Can you work these out from the model? Positions are in its coordinate system, mm. Round coordinates to 2 decimals unless told otherwise and drop trailing zeros. Loops run counter-clockwise (first coordinate to the right, second up) from the corner with the lowest first, then second, coordinate; pieces in that order, holes last. Notation, with made-up numbers: M 13,88 L 58,88 A20 cw 58,102 Z; hole C -35,46.25 d8. An arc over 180 degrees is marked long. Return JSON: item names as keys, results as strings.
```python
from build123d import *

# Parameters (mm, degrees)
ESQUISSE1_R        = 6.75
ESQUISSE1_R_2      = 41.5
ESQUISSE1_W        = 40
ESQUISSE1_H        = 80
BOSS_EXTRU_1_DEPTH = 10
CONG_1_R           = 10


with BuildPart() as part:
    # Esquisse1 → Boss.-Extru.1 (new body)
    with BuildSketch(Plane(origin=(0, 0, 0), x_dir=(0, 0, -1), z_dir=(1, 0, 0))):
        with BuildLine():
            ThreePointArc((229.796105276, 60), (0, 237.5), (-229.796105276, 60))
            ThreePointArc((-229.796105276, 60), (-231.618451309, 52.527545282), (-233.197877349, 45))
            ThreePointArc((-233.197877349, 45), (-237.5, 0), (-233.197877349, -45))
            ThreePointArc((-233.197877349, -45), (-231.618451309, -52.527545282), (-229.796105276, -60))
            ThreePointArc((-229.796105276, -60), (0, -237.5), (229.796105276, -60))
            ThreePointArc((229.796105276, -60), (231.618451309, -52.527545282), (233.197877349, -45))
            ThreePointArc((233.197877349, -45), (236.422022949, -22.602589781), (237.5, 0))
            ThreePointArc((237.5, 0), (236.422022949, 22.602589781), (233.197877349, 45))
            ThreePointArc((233.197877349, 45), (231.618451309, 52.527545282), (229.796105276, 60))
        make_face()
        with Locations((-158.391918986, -158.391918986)):
            Circle(ESQUISSE1_R, mode=Mode.SUBTRACT)
        with Locations((-85.72108885, -206.949015283)):
            Circle(ESQUISSE1_R, mode=Mode.SUBTRACT)
        with Locations((-206.949015283, -85.72108885)):
            Circle(ESQUISSE1_R, mode=Mode.SUBTRACT)
        with Locations((-224, 0)):
            Circle(ESQUISSE1_R, mode=Mode.SUBTRACT)
        with Locations((-53, -98.5)):
            Circle(ESQUISSE1_R, mode=Mode.SUBTRACT)
        with Locations((0, -224)):
            Circle(ESQUISSE1_R, mode=Mode.SUBTRACT)
        with Locations((85.72108885, -206.949015283)):
            Circle(ESQUISSE1_R, mode=Mode.SUBTRACT)
        with Locations((158.391918986, -158.391918986)):
            Circle(ESQUISSE1_R, mode=Mode.SUBTRACT)
        with Locations((0, -98.5)):
            Circle(ESQUISSE1_R_2, mode=Mode.SUBTRACT)
        with Locations((53, -98.5)):
            Circle(ESQUISSE1_R, mode=Mode.SUBTRACT)
        with Locations((206.949015283, -85.72108885)):
            Circle(ESQUISSE1_R, mode=Mode.SUBTRACT)
        with Locations((-150, 0)):
            Rectangle(ESQUISSE1_W, ESQUISSE1_H, mode=Mode.SUBTRACT)
        with Locations((-206.949015283, 85.72108885)):
            Circle(ESQUISSE1_R, mode=Mode.SUBTRACT)
        with BuildLine():
            Line((-20, 60), (-159.059737206, 60))
            ThreePointArc((-159.059737206, 60), (-104.766475875, 133.880489739), (-20, 168.819430161))
            Line((-20, 168.819430161), (-20, 60))
        make_face(mode=Mode.SUBTRACT)
        with Locations((-158.391918986, 158.391918986)):
            Circle(ESQUISSE1_R, mode=Mode.SUBTRACT)
        with Locations((-85.72108885, 206.949015283)):
            Circle(ESQUISSE1_R, mode=Mode.SUBTRACT)
        with BuildLine():
            Line((159.059737206, 60), (20, 60))
            Line((20, 60), (20, 168.819430161))
            ThreePointArc((20, 168.819430161), (104.766475875, 133.880489739), (159.059737206, 60))
        make_face(mode=Mode.SUBTRACT)
        with Locations((150, 0)):
            Rectangle(ESQUISSE1_W, ESQUISSE1_H, mode=Mode.SUBTRACT)
        with Locations((224, 0)):
            Circle(ESQUISSE1_R, mode=Mode.SUBTRACT)
        with Locations((206.949015283, 85.72108885)):
            Circle(ESQUISSE1_R, mode=Mode.SUBTRACT)
        with Locations((0, 224)):
            Circle(ESQUISSE1_R, mode=Mode.SUBTRACT)
        with Locations((85.72108885, 206.949015283)):
            Circle(ESQUISSE1_R, mode=Mode.SUBTRACT)
        with Locations((158.391918986, 158.391918986)):
            Circle(ESQUISSE1_R, mode=Mode.SUBTRACT)
    extrude(amount=BOSS_EXTRU_1_DEPTH)

    # Cong_1
    cong_1_edges = [part.edges().sort_by_distance(p)[0] for p in [
        (5, 60, -20),
        (5, 60, -159.059737206),
        (5, 168.819430161, -20),
        (5, 60, 159.059737206),
        (5, 60, 20),
        (5, 168.819430161, 20),
    ]]
    fillet(cong_1_edges, radius=CONG_1_R)


solid = part.part
```
Q1. Suppose I cut it at B-B, the plane y = -224. Please give me the cut outline in (x, z).
Results:
{"outline": "M 0,-78.93 L 10,-78.93 L 10,-6.75 L 0,-6.75 Z; M 0,6.75 L 10,6.75 L 10,78.93 L 0,78.93 Z"}
Q2. Suppose I cut it at C-C, the plane z = 53. Please give me the cut outline in (x, y), plus the area to 3 significant figures.
Results:
{"outline": "M 0,-231.51 L 10,-231.51 L 10,-105.25 L 0,-105.25 Z; M 0,-91.75 L 10,-91.75 L 10,60 L 0,60 Z; M 0,161.53 L 10,161.53 L 10,231.51 L 0,231.51 Z", "area": "3,480 mm2"}
Q3. Suppose I cut it at A-A, the plane z = 0. Please give me the cut outline in (x, y), plus the area to 3 significant figures.
Results:
{"outline": "M 0,-237.5 L 10,-237.5 L 10,-230.75 L 0,-230.75 Z; M 0,-217.25 L 10,-217.25 L 10,-140 L 0,-140 Z; M 0,-57 L 10,-57 L 10,217.25 L 0,217.25 Z; M 0,230.75 L 10,230.75 L 10,237.5 L 0,237.5 Z", "area": "3,650 mm2"}
Q4. If I drill on line 1 along Z through (x, y) = (7.25, 34); line 2 along Z through (x, y) = (9.25, 90.5); line 3 along Z through (x, y) = (3, 9), over which ranges is the centre line in solid material (lowest first)?
Results:
{"line 1": "z = -235.05 to -170, -130 to 130, 170 to 235.05", "line 2": "z = -219.58 to -211.72, -202.18 to -143.91, -20 to 20, 143.91 to 202.18, 211.72 to 219.58", "line 3": "z = -237.33 to -170, -130 to 130, 170 to 237.33"}
Q5. I'm going to push flat-ended pins straight in: pin 1 Ø2 at (x, y) = (4, -159) entering from -Z; pin 2 Ø1 at (x, z) = (2, -122.5) entering from +Y; pin 3 Ø6 at (x, y) = (7, 101.5) entering from +Z. Where does each tip first touch, or does it pass through?
Results:
{"pin 1": "stops at z = -177.32", "pin 2": "stops at y = 203.77", "pin 3": "stops at z = 216.11"}
Q6. Suppose I cut it at D-D, the plane y = -25. Please give me the cut outline in (x, z).
Results:
{"outline": "M 0,-236.18 L 10,-236.18 L 10,-170 L 0,-170 Z; M 0,-130 L 10,-130 L 10,130 L 0,130 Z; M 0,170 L 10,170 L 10,236.18 L 0,236.18 Z"}
Q7. Thinking about a two-plate mould opening in Z: for faces 1 (the cylindrical face through (4.93, -158.1, -151.65)), 2 (the flat face through (0, 3, 3)), which applies, pulls with the +Z half, pulls with the -Z half, needs draft (parallel to the pull), parting line crosses it, or undercut?
Results:
{"face 1": "undercut", "face 2": "needs draft"}
